Check sheet for the modelled part. Datum: model origin and axes. Units: mm. Face numbers are marked on the shaded views. A direction names the side the tool comes from. Coordinates: 2 decimals unless noted, no trailing zeros. Loops run counter-clockwise (first coordinate to the right, second up) from the corner with the lowest first, then second, coordinate; pieces in that order, holes last. Notation, with made-up numbers: (77.5, -1) - (98.5, -1) arc R11 cw to (98.5, 8) - close; hole circle Ø2 at (1.5, 68.25). An arc over 180 degrees is marked (long way). Use a Markdown table: item, result. Add a question column.
1) Sectioned sample at C-C, the plane z = 10.5. Enter the section's corners in (x, y) (3 decimals), then the cut area to 3 significant figures.
2) Thickness scan on line 1 (Z direction, x = -9.75, y = -4.75) (3 decimals); line 2 (Y direction, x = 3.75, z = 1.5); line 3 (Y direction, x = 4.75, z = 10.25). Record the ranges inside material, lowest first.
3) Tool access check on the marked faces 1 and 2. Record the directions out of +Z, -Z, +X, -X, +Y, -Y that give a thin tool (end or side, any length) a straight path to the whole face; none if there is none.
4) Sectioned sample at D-D, the plane z = 8.5. Enter the section's corners in (x, y) (1 decimal), then the cut area to 3 significant figures.
5) Go/stop test with flat-tipped pins: P1, Ø5, axis at x = -9, z = 6.5, coming from the +Y side; P2, Ø1.5, axis at y = 2, z = 10.5, coming from the +X side. Record where each tip stops, or that it passes through.
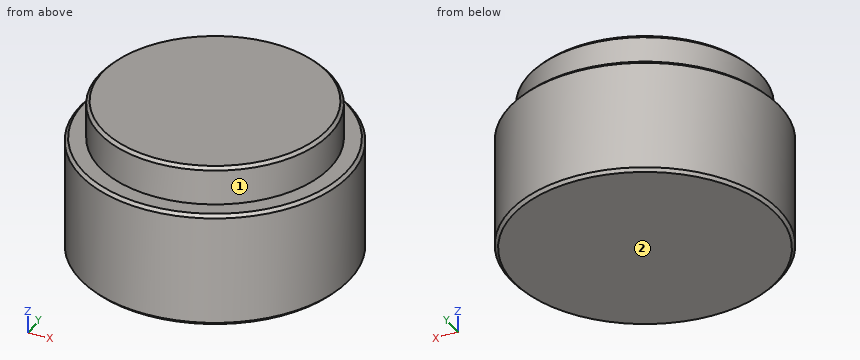
Autodesk Inventor part; units mm, degrees
ref_plane "YZ Plane" through (0, 0, 0) normal (1, 0, 0) x (0, 1, 0)
ref_plane "XZ Plane" through (0, 0, 0) normal (0, 1, 0) x (-1, 0, 0)
ref_plane "XY Plane" through (0, 0, 0) normal (0, 0, 1) x (1, 0, 0)
sketch "Sketch1" plane through (0, 0, 0) normal (0, 0, 1) x (1, 0, 0)
  circle A0 centre (0, 0) radius 11.1125
  dimension "d5" = 22.225
extrude "Extrusion1" add sketch "Sketch1" along normal blind 9.525
sketch "Sketch2" plane through (0, 0, 9.525) normal (0, 0, 1) x (1, 0, 0)
  circle A0 centre (0, 0) radius 11.1125
  circle A1 centre (0, 0) radius 9.525
  dimension "d4" = 19.05
extrude "Extrusion2" add sketch "Sketch2" along normal blind 3.175 contours A1
chamfer "Chamfer1" distance 0.254 angle 45 3 edges at (-9.525, 0, 12.7) (-11.1125, 0, 9.525) (-11.1125, 0, 0)
properties part number "rear cyl head"
Solved:
| question | item | result |
|---|---|---|
| 1 | outline | circle Ø19.05 at (0, 0) |
| 1 | area | 285 mm2 |
| 2 | line 1 | z = 0 to 9.525 |
| 2 | line 2 | y = -10.46 to 10.46 |
| 2 | line 3 | y = -8.26 to 8.26 |
| 3 | face 1 | +Z |
| 3 | face 2 | -Z, +X, -X, +Y, -Y |
| 4 | outline | circle Ø22.2 at (0, 0) |
| 4 | area | 388 mm2 |
| 5 | P1 | stops at y = 9.01 |
| 5 | P2 | stops at x = 9.44 |
